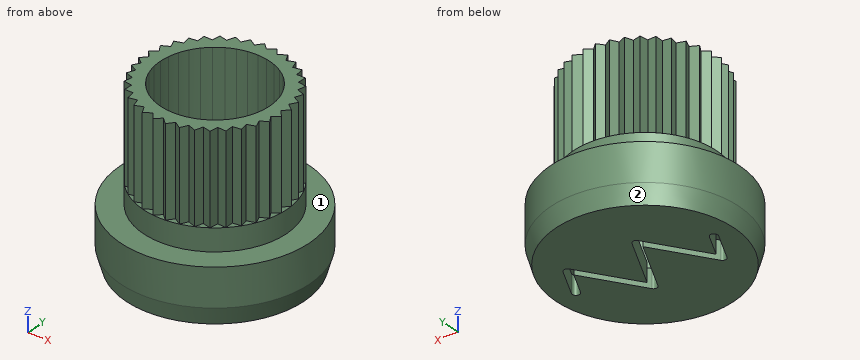
from build123d import *

# Parameters (mm, degrees)
PAD_DEPTH          = 12
POLARPATTERN_COUNT = 36
SKETCH001_R        = 9.64
SKETCH001_R_2      = 7.35
PAD001_DEPTH       = 3
SKETCH002_R        = 12.7
SKETCH002_R_2      = 7.35
PAD002_DEPTH       = 5
SKETCH003_R        = 12.7
PAD003_DEPTH       = 2.5
CHAMFER_SIZE2      = 0.7
CHAMFER_SIZE       = 2.4


with BuildPart() as part:
    # Sketch → Pad (new body)
    with BuildSketch(Plane.XY):
        with BuildLine():
            Line((0, 8.85), (0.8401813601, 9.6033168896))
            Line((1.5367863724, 8.7155486142), (0.8401813601, 9.6033168896))
            Line((1.2763141059, 7.2383369846), (1.5367863724, 8.7155486142))
            ThreePointArc((1.2763141059, 7.2383369846), (0.6405947092, 7.322031031), (0, 7.35))
            Line((0, 7.35), (0, 8.85))
        make_face()
    pad = extrude(amount=PAD_DEPTH)

    # PolarPattern: Pad ×36 about axis
    polarpattern_axis = Axis((0, 0, 0), (0, 0, 1))
    for i in range(1, POLARPATTERN_COUNT):
        add(pad.rotate(polarpattern_axis, i * 360 / POLARPATTERN_COUNT))

    # Sketch001 (on DatumPlane) → Pad001 (join)
    with BuildSketch(Plane.XY):
        Circle(SKETCH001_R)
        Circle(SKETCH001_R_2, mode=Mode.SUBTRACT)
    extrude(amount=-PAD001_DEPTH)

    # Sketch002 (on Face51 of Pad001) → Pad002 (join)
    with BuildSketch(Plane(origin=(0, 0, -3), x_dir=(1, 0, 0), z_dir=(0, 0, -1))):
        Circle(SKETCH002_R)
        Circle(SKETCH002_R_2, mode=Mode.SUBTRACT)
    extrude(amount=PAD002_DEPTH)

    # Sketch003 (on DatumPlane) → Pad003 (join)
    with BuildSketch(Plane(origin=(0, 0, -8), x_dir=(1, 0, 0), z_dir=(0, 0, -1))):
        Circle(SKETCH003_R)
        with BuildLine():
            ThreePointArc((-9.7272135955, 0.2236067977), (-9.5036067977, -0.4472135955), (-8.8327864045, -0.2236067977))
            Line((-8.8327864045, -0.2236067977), (-7.2200847391, 3.001796533))
            Line((-2.4152236623, -4.2754949357), (-7.2200847391, 3.001796533))
            ThreePointArc((-2.4152236623, -4.2754949357), (-1.9680100668, -4.4991017335), (-1.5507541017, -4.2236067977))
            Line((-1.5507541017, -4.2236067977), (2.061789241, 3.0014798877))
            Line((2.061789241, 3.0014798877), (6.8626465602, -4.2753472467))
            ThreePointArc((6.8626465602, -4.2753472467), (7.309869311, -4.4991070269), (7.7272135955, -4.2236067977))
            Line((7.7272135955, -4.2236067977), (9.7272135955, -0.2236067977))
            ThreePointArc((9.7272135955, -0.2236067977), (9.5036067977, 0.4472135955), (8.8327864045, 0.2236067977))
            Line((7.2202430618, -3.0014798877), (8.8327864045, 0.2236067977))
            Line((2.4193857426, 4.2753472467), (7.2202430618, -3.0014798877))
            ThreePointArc((2.4193857426, 4.2753472467), (1.9721629918, 4.4991070269), (1.5548187073, 4.2236067977))
            Line((-2.0578829581, -3.001796533), (1.5548187073, 4.2236067977))
            Line((-6.8627440349, 4.2754949357), (-2.0578829581, -3.001796533))
            ThreePointArc((-6.8627440349, 4.2754949357), (-7.3099576304, 4.4991017335), (-7.7272135955, 4.2236067977))
            Line((-9.7272135955, 0.2236067977), (-7.7272135955, 4.2236067977))
        make_face(mode=Mode.SUBTRACT)
    extrude(amount=PAD003_DEPTH)

    # Chamfer
    chamfer_edges = [part.edges().sort_by_distance(p)[0] for p in [
        (-12.7, 0, -10.5),
    ]]
    chamfer_side = part.faces().sort_by_distance((-12.7, 0, -9.25))[0]
    chamfer(chamfer_edges, length=CHAMFER_SIZE, length2=CHAMFER_SIZE2, reference=chamfer_side)


solid = part.part
Check sheet for the modelled part. Datum: model origin and axes. Units: mm. Face numbers are marked on the shaded views. A direction names the side the tool comes from. Coordinates: 2 decimals unless noted, no trailing zeros. Write each loop counter-clockwise with the first axis right and the second up, starting at its lowest first coordinate (ties: lowest second). Pieces come first, ordered by that corner, then holes.
Item 1: Access from +Z, -Z, +X, -X, +Y, -Y to the whole of each face (thin tool, end or side, straight path). Record for the marked faces 1 and 2.
Numbers:
face 1: +Z
face 2: -Z
Item 2: Cross-section at A-A on z = -6.5. Record the boundary of the cut face in (x, y), then the cut area to 3 significant figures.
Numbers:
outline: circle Ø25.4 at (0, 0); hole circle Ø14.7 at (0, 0)
area: 337 mm2
Item 3: Scan lines: probe 1 along X at (y, z) = (0, -5.05); probe 2 along Y at (x, z) = (0, -0.8). Record each from-to range of solid material in increasing order.
Numbers:
probe 1: x = -12.7 to -7.35, 7.35 to 12.7
probe 2: y = -9.64 to -7.35, 7.35 to 9.64
Item 4: Depth check by flat-ended pin: pin 1 Ø12 at (y, z) = (5, -4.5) entering from -X; pin 2 Ø1.5 at (x, y) = (-4.5, 3.5) entering from +Z; pin 3 Ø6 at (x, z) = (-10, 4) entering from +Y; pin 4 Ø0.6 at (x, y) = (0, -9.5) entering from +Z. Enter the tip coordinate at first touch or a pass-through.
Numbers:
pin 1: stops at x = -12.7
pin 2: stops at z = -8
pin 3: stops at y = 5.66
pin 4: stops at z = 0
